Design review of the part built by this model. Coordinates are the model's own, in mm. Face numbers are marked on the shaded views. A direction names the side the tool comes from. Give positions to 0.01 mm unless a question says otherwise; leave off trailing zeros. Loops run counter-clockwise (first coordinate to the right, second up) from the corner with the lowest first, then second, coordinate; pieces in that order, holes last. Notation, with made-up numbers: (-28.5, 52.25) - (7.5, 52.25) arc R25 cw to (7.5, 84.25) - close; hole circle Ø7 at (47.25, 4.25). An arc over 180 degrees is marked (long way). Write each question's results on one line, items separated by ' | '.
```python
from build123d import *

# Parameters (mm, degrees)
SKETCH1_W           = 16
SKETCH1_H           = 40
BOSS_EXTRUDE1_DEPTH = 40
SKETCH2_W           = 16
SKETCH2_H           = 3.7
BOSS_EXTRUDE2_DEPTH = 16
SKETCH5_W           = 10
SKETCH5_H           = 34
CUT_EXTRUDE3_DEPTH  = 37
FILLET1_R           = 1
FILLET2_R           = 1
CUT_EXTRUDE6_DEPTH  = 3.5
SKETCH9_W           = 16
SKETCH9_H           = 1
BOSS_EXTRUDE3_DEPTH = 2
CUT_EXTRUDE7_REACH  = 61.78
SKETCH12_R          = 2.1
CUT_EXTRUDE8_REACH  = 50.884
SKETCH13_R          = 2.1
FILLET3_R           = 2


with BuildPart() as part:
    # Sketch1 → Boss-Extrude1 (new body)
    with BuildSketch(Plane(origin=(0, 0, 0), x_dir=(1, 0, 0), z_dir=(0, 1, 0))):
        Rectangle(SKETCH1_W, SKETCH1_H)
    extrude(amount=BOSS_EXTRUDE1_DEPTH)

    # Sketch2 → Boss-Extrude2 (add)
    with BuildSketch(Plane.XZ):
        with Locations((0, 21.85)):
            Rectangle(SKETCH2_W, SKETCH2_H)
        with Locations((0, -21.85)):
            Rectangle(SKETCH2_W, SKETCH2_H)
    extrude(amount=-BOSS_EXTRUDE2_DEPTH)

    # Sketch5 → Cut-Extrude3 (cut)
    with BuildSketch(Plane.XZ):
        Rectangle(SKETCH5_W, SKETCH5_H)
    extrude(amount=-CUT_EXTRUDE3_DEPTH, mode=Mode.SUBTRACT)

    # Fillet1
    fillet1_edges = [part.edges().sort_by_distance(p)[0] for p in [
        (8, 40, 0),
        (0, 40, -20),
        (-8, 16, 21.85),
        (8, 16, 21.85),
        (0, 16, 20),
        (-8, 16, -21.85),
        (0, 16, -20),
        (8, 16, -21.85),
        (-8, 40, 0),
        (0, 40, 20),
        (-8, 28, -20),
        (8, 28, -20),
        (8, 28, 20),
        (-8, 28, 20),
    ]]
    fillet(fillet1_edges, radius=FILLET1_R)

    # Fillet2
    fillet2_edges = [part.edges().sort_by_distance(p)[0] for p in [
        (-5, 37, 0),
        (-5, 18.5, -17),
        (0, 37, 17),
        (-5, 18.5, 17),
        (5, 37, 0),
        (5, 18.5, 17),
        (0, 37, -17),
        (5, 18.5, -17),
    ]]
    fillet(fillet2_edges, radius=FILLET2_R)

    # Sketch3 → Cut-Extrude6 (cut)
    with BuildSketch(Plane(origin=(0, 0, -23.7), x_dir=(-1, 0, 0), z_dir=(0, 0, -1))):
        Polygon((2.078460969, 11.6), (-2.078460969, 11.6), (-4.156921938, 8), (-2.078460969, 4.4), (2.078460969, 4.4), (4.156921938, 8), align=None)
    cut_extrude6 = extrude(amount=-CUT_EXTRUDE6_DEPTH, mode=Mode.SUBTRACT)

    # Mirror2: Cut-Extrude6 across plane
    add(cut_extrude6.mirror(Plane.XY), mode=Mode.SUBTRACT)

    # Sketch9 → Boss-Extrude3 (add)
    with BuildSketch(Plane.XZ):
        with Locations((0, 20.7)):
            Rectangle(SKETCH9_W, SKETCH9_H)
        with Locations((0, -20.7)):
            Rectangle(SKETCH9_W, SKETCH9_H)
    extrude(amount=BOSS_EXTRUDE3_DEPTH)

    # Sketch12 → Cut-Extrude7 (cut, up to next)
    with BuildSketch(Plane.XY.offset(20), mode=Mode.PRIVATE) as cut_extrude7_sk1:
        with Locations((0, 24)):
            Circle(SKETCH12_R)
    cut_extrude7_tool1 = extrude(cut_extrude7_sk1.sketch, amount=-CUT_EXTRUDE7_REACH, mode=Mode.PRIVATE) & part.part
    add(cut_extrude7_tool1.solids().sort_by_distance((0, 24, 20))[0], mode=Mode.SUBTRACT)

    # Sketch13 → Cut-Extrude8 (cut, up to next)
    with BuildSketch(Plane(origin=(0, 40, 0), x_dir=(1, 0, 0), z_dir=(0, 1, 0)), mode=Mode.PRIVATE) as cut_extrude8_sk1:
        with Locations(Location((0, 10, 0), (0, 0, 270))):
            Circle(SKETCH13_R)
    cut_extrude8_tool1 = extrude(cut_extrude8_sk1.sketch, amount=-CUT_EXTRUDE8_REACH, mode=Mode.PRIVATE) & part.part
    add(cut_extrude8_tool1.solids().sort_by_distance((0, 40, -10))[0], mode=Mode.SUBTRACT)

    # Fillet3
    fillet3_edges = [part.edges().sort_by_distance(p)[0] for p in [
        (0, 0, 21.2),
        (0, 0, -21.2),
    ]]
    fillet(fillet3_edges, radius=FILLET3_R - 0.0001)  # a hair under: the kernel refuses the full size


solid = part.part
```
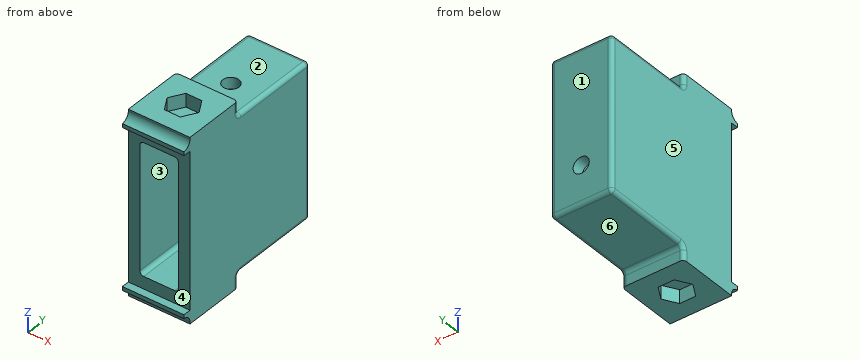
Item 1: We need section D-D on y = 24. Give the boundary of the cut face in (x, z).
Output values:
outline: (-8, -19) arc R1 ccw to (-7, -20) - (7, -20) arc R1 ccw to (8, -19) - (8, 19) arc R1 ccw to (7, 20) - (2.1, 20) - (2.1, 17) - (4, 17) arc R1 cw to (5, 16) - (5, -16) arc R1 cw to (4, -17) - (-4, -17) arc R1 cw to (-5, -16) - (-5, 16) arc R1 cw to (-4, 17) - (-2.1, 17) - (-2.1, 20) - (-7, 20) arc R1 ccw to (-8, 19) - close
Item 2: We need section B-B on y = 13. Give the boundary of the cut face in (x, z).
Output values:
outline: (-8, -23.7) - (8, -23.7) - (8, 23.7) - (-8, 23.7) - close; hole (-5, -16) arc R1 ccw to (-4, -17) - (4, -17) arc R1 ccw to (5, -16) - (5, 16) arc R1 ccw to (4, 17) - (-4, 17) arc R1 ccw to (-5, 16) - close
Item 3: Tool access review of the marked faces 1, 2 and 3: name each direction out of +Z, -Z, +X, -X, +Y, -Y from which nothing blocks a thin tool from reaching the whole face with its end or side.
Output values:
face 1: +Z, -Z, +X, -X, +Y | face 2: +Z, +X, -X, +Y | face 3: -Y
Item 4: We need section A-A on z = -10. Give the boundary of the cut face in (x, y).
Output values:
outline: (-8, 0) - (-5, 0) - (-5, 36) arc R1 cw to (-4, 37) - (-2.1, 37) - (-2.1, 40) - (-7, 40) arc R1 ccw to (-8, 39) - close; (2.1, 37) - (4, 37) arc R1 cw to (5, 36) - (5, 0) - (8, 0) - (8, 39) arc R1 ccw to (7, 40) - (2.1, 40) - close
Item 5: Clearance check with flat-ended pins moving along their axes: P1, Ø7, axis at x = 1.5, y = 32, coming from the +Z side; P2, Ø1, axis at x = -0.5, y = -1, coming from the -Z side; P3, Ø1, axis at x = 3, y = 22.5, coming from the -Z side. State where each tip first meets the part, or that it passes through.
Output values:
P1: stops at z = 20 | P2: stops at z = -21.88 | P3: stops at z = -20
Item 6: Wall thickness on probe 1 along Z at (x, y) = (0.75, 26); probe 2 along X at (y, z) = (9, -13.5); probe 3 along Z at (x, y) = (2.25, 12): over which ranges is each line inside the solid? List them lowest first.
Output values:
probe 1: z = -20 to -17, 17 to 20 | probe 2: x = -8 to -5, 5 to 8 | probe 3: z = -23.7 to -17, 17 to 23.7
Item 7: We need section C-C on z = 1. Give the boundary of the cut face in (x, y).
Output values:
outline: (-8, 0) - (-5, 0) - (-5, 36) arc R1 cw to (-4, 37) - (4, 37) arc R1 cw to (5, 36) - (5, 0) - (8, 0) - (8, 39) arc R1 ccw to (7, 40) - (-7, 40) arc R1 ccw to (-8, 39) - close
Item 8: Draft analysis for pull direction Z (two halves, no side actions). For the marked faces 4, 5 and 6, state which applies: +Z half, -Z half, draft (parallel to the pull), parting line (faces both ways), or undercut.
Output values:
face 4: undercut | face 5: draft | face 6: -Z half
